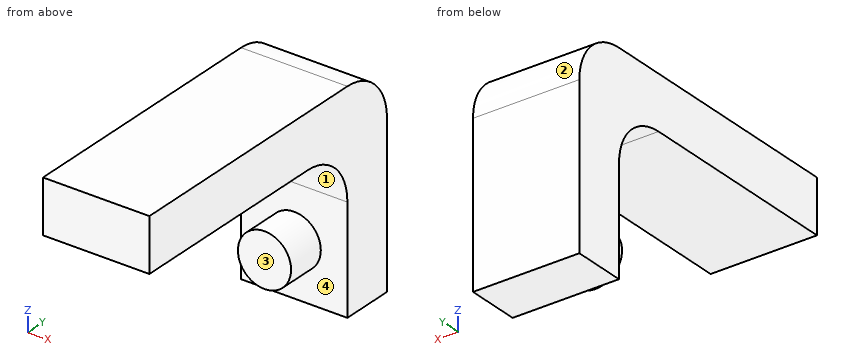
from build123d import *

# Parameters (mm, degrees)
SALIENTE_EXTRUIR1_DEPTH = 50.8
CROQUIS2_R              = 12.7
SALIENTE_EXTRUIR2_DEPTH = 19.05


with BuildPart() as part:
    # Croquis1 → Saliente-Extruir1 (new body)
    with BuildSketch(Plane(origin=(0, 0, 0), x_dir=(0, 0, -1), z_dir=(1, 0, 0))):
        with BuildLine():
            Line((0, 0), (25.4, 0))
            Line((25.4, 0), (25.4, 101.6))
            ThreePointArc((25.4, 101.6), (32.839487758, 119.560512242), (50.8, 127))
            Line((50.8, 127), (101.6, 127))
            Line((101.6, 127), (101.6, 152.4))
            Line((101.6, 152.4), (25.4, 152.4))
            ThreePointArc((25.4, 152.4), (7.439487758, 144.960512242), (0, 127))
            Line((0, 127), (0, 0))
        make_face()
    extrude(amount=SALIENTE_EXTRUIR1_DEPTH)

    # Croquis2 → Saliente-Extruir2 (add)
    with BuildSketch(Plane.XZ.offset(-127)):
        with Locations((25.4, -76.2)):
            Circle(CROQUIS2_R)
    extrude(amount=SALIENTE_EXTRUIR2_DEPTH)


solid = part.part
Input: part model. Units: mm. Frame: model coordinates. Face numbers are marked on the shaded views. A direction names the side the tool comes from. Coordinates: 2 decimals unless noted, no trailing zeros. Order: outer loops, then holes, each group sorted by start corner. A loop starts at its lowest first (then second) coordinate and runs counter-clockwise, first axis right, second up.
1. Cut plane B-B, the plane z = -76.2. Return loops of the section in (x, y), plus the area to 3 significant figures.
Checked values:
outline: (0, 127) - (12.7, 127) - (12.7, 107.95) - (38.1, 107.95) - (38.1, 127) - (50.8, 127) - (50.8, 152.4) - (0, 152.4) - close
area: 1,770 mm2
2. Contact query for flat-ended pins moving along their axis: P1, Ø5, axis at x = 34.5, y = 61, coming from the -Z side; P2, Ø2, axis at y = 110.5, z = -73.5, coming from the +X side; P3, Ø10, axis at x = 26, z = -59, coming from the -Y side. Output: stop coordinate, or through.
Checked values:
P1: stops at z = -25.4
P2: stops at x = 37.99
P3: stops at y = 107.95
3. Cut plane A-A, the plane x = 25.4. Return loops of the section in (y, z).
Checked values:
outline: (0, -25.4) - (101.6, -25.4) arc R25.4 cw to (127, -50.8) - (127, -63.5) - (107.95, -63.5) - (107.95, -88.9) - (127, -88.9) - (127, -101.6) - (152.4, -101.6) - (152.4, -25.4) arc R25.4 ccw to (127, 0) - (0, 0) - close
4. Cut plane C-C, the plane y = 41.5. Return loops of the section in (x, z), plus the area to 3 significant figures.
Checked values:
outline: (0, -25.4) - (50.8, -25.4) - (50.8, 0) - (0, 0) - close
area: 1,290 mm2
5. Cut plane D-D, the plane x = 10. Return loops of the section in (y, z), plus the area to 3 significant figures.
Checked values:
outline: (0, -25.4) - (101.6, -25.4) arc R25.4 cw to (127, -50.8) - (127, -101.6) - (152.4, -101.6) - (152.4, -25.4) arc R25.4 ccw to (127, 0) - (0, 0) - close
area: 5,810 mm2
6. Ray query, line 1 along Y through (x, z) = (2.5, -71); line 2 along Z through (x, y) = (44.5, 50.5); line 3 along Y through (x, z) = (22, -71). Return the intervals inside material, ascending.
Checked values:
line 1: y = 127 to 152.4
line 2: z = -25.4 to 0
line 3: y = 107.95 to 152.4
7. Access query for the marked faces 1, 2, 3 and 4. Directions: +Z, -Z, +X, -X, +Y, -Y. A direction counts if a zero-diameter tool reaches every point of the face in a straight line with its end or side. Return the directions, or none.
Checked values:
face 1: +X, -X, -Y
face 2: +Z, +X, -X, +Y
face 3: -Z, +X, -X, -Y
face 4: -Y
